from build123d import *

# Parameters (mm, degrees)
SKETCH_1_R      = 1.65
SKETCH_1_R_2    = 1.4
SKETCH_1_R_3    = 1.5
EXTRUDE_1_DEPTH = 4


with BuildPart() as part:
    # 草图1 → 凸台-拉伸1 (new body)
    with BuildSketch(Plane.XY):
        with BuildLine():
            ThreePointArc((-3.477620962, -15.10483871), (0, -19), (3.477620962, -15.10483871))
            ThreePointArc((3.477620962, -15.10483871), (6.883154194, -6.883154194), (15.10483871, -3.477620962))
            ThreePointArc((15.10483871, -3.477620962), (19, 0), (15.10483871, 3.477620962))
            ThreePointArc((15.10483871, 3.477620962), (6.883154194, 6.883154194), (3.477620962, 15.10483871))
            ThreePointArc((3.477620962, 15.10483871), (0, 19), (-3.477620962, 15.10483871))
            ThreePointArc((-3.477620962, 15.10483871), (-6.883154194, 6.883154194), (-15.10483871, 3.477620962))
            ThreePointArc((-15.10483871, 3.477620962), (-19, 0), (-15.10483871, -3.477620962))
            ThreePointArc((-15.10483871, -3.477620962), (-6.883154194, -6.883154194), (-3.477620962, -15.10483871))
        make_face()
        Circle(SKETCH_1_R, mode=Mode.SUBTRACT)
        with Locations((0, -6.5)):
            Circle(SKETCH_1_R_2, mode=Mode.SUBTRACT)
        with Locations((0, 6.5)):
            Circle(SKETCH_1_R_2, mode=Mode.SUBTRACT)
        with Locations((0, -15.5)):
            Circle(SKETCH_1_R_3, mode=Mode.SUBTRACT)
        with Locations((-15.5, 0)):
            Circle(SKETCH_1_R_3, mode=Mode.SUBTRACT)
        with Locations((0, 15.5)):
            Circle(SKETCH_1_R_3, mode=Mode.SUBTRACT)
        with Locations((15.5, 0)):
            Circle(SKETCH_1_R_3, mode=Mode.SUBTRACT)
    extrude(amount=EXTRUDE_1_DEPTH)


solid = part.part
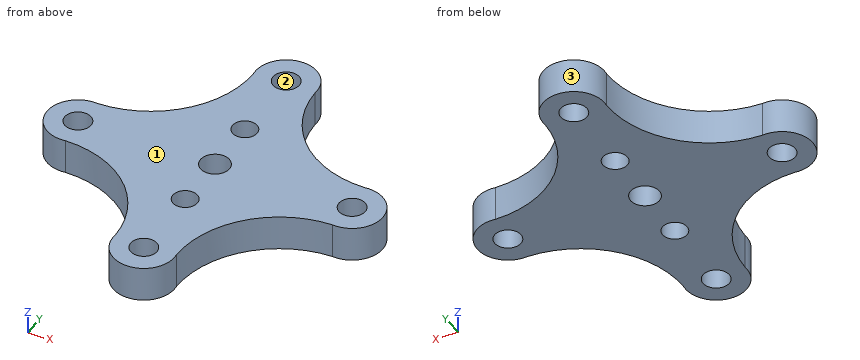
Could you check a few things on this model? Use its own coordinates, in mm. Face numbers are marked on the shaded views. Give positions to 0.01 mm unless a question says otherwise; leave off trailing zeros. Write each loop counter-clockwise with the first axis right and the second up, starting at its lowest first coordinate (ties: lowest second). Pieces come first, ordered by that corner, then holes. Notation, with made-up numbers: (14, 33.25) -> (21, 33.25) arc R14 cw to (21, 55.25) -> close; hole circle Ø7 at (49, 8). An arc over 180 degrees is marked (long way). Answer as CSV lines item,"result". Start each with the question number.
(1) Please list where these lines run through material, in increasing order: line 1 (Y direction, x = 0, z = 2.05); line 2 (X direction, y = -16, z = 0.95); line 3 (X direction, y = 4.5, z = 0.3).
(2) If we section it at B-B, the plane y = 0: Write out the boundary of the cut face in (x, z).
(3) If we section it at C-C, the plane z = 0.85: Write out the boundary of the cut face in (x, y).
(4) If we section it at D-D, the plane y = 6: Write out the boundary of the cut face in (x, z).
(5) I'm going to push flat-ended pins straight in: pin 1 Ø2.5 at (x, y) = (15.5, 0) entering from +Z; pin 2 Ø2 at (y, z) = (-2, 3) entering from -X. Where does each tip first touch, or does it pass through?
(6) If we mould it in two halves opening along X, with no side actions, what happens to the marked faces 1, 2 and 3? For each: +X half, -X half, draft (parallel to the pull), parting line (faces both ways), or undercut.
(7) If we section it at A-A, the plane y = -6.5: Write out the boundary of the cut face in (x, z), and give its area (3 significant figures).
Answer list:
1,line 1,"-19 to -17, -14 to -7.9, -5.1 to -1.65, 1.65 to 5.1, 7.9 to 14, 17 to 19"
1,line 2,"-3.46 to -1.41, 1.41 to 3.46"
1,line 3,"-10.34 to 10.34"
2,outline,"(-19, 0) -> (-17, 0) -> (-17, 4) -> (-19, 4) -> close; (-14, 0) -> (-1.65, 0) -> (-1.65, 4) -> (-14, 4) -> close; (1.65, 0) -> (14, 0) -> (14, 4) -> (1.65, 4) -> close; (17, 0) -> (19, 0) -> (19, 4) -> (17, 4) -> close"
3,outline,"(-15.1, -3.48) arc R11.63 cw to (-3.48, -15.1) arc R3.5 ccw (long way) to (3.48, -15.1) arc R11.63 cw to (15.1, -3.48) arc R3.5 ccw (long way) to (15.1, 3.48) arc R11.63 cw to (3.48, 15.1) arc R3.5 ccw (long way) to (-3.48, 15.1) arc R11.63 cw to (-15.1, 3.48) arc R3.5 ccw (long way) to start; hole circle Ø3 at (-15.5, 0); hole circle Ø3.3 at (0, 0); hole circle Ø3 at (0, -15.5); hole circle Ø3 at (0, 15.5); hole circle Ø2.8 at (0, -6.5); hole circle Ø2.8 at (0, 6.5); hole circle Ø3 at (15.5, 0)"
4,outline,"(-7.87, 0) -> (-1.31, 0) -> (-1.31, 4) -> (-7.87, 4) -> close; (1.31, 0) -> (7.87, 0) -> (7.87, 4) -> (1.31, 4) -> close"
5,pin 1,"through"
5,pin 2,"x = -18.85"
6,face 1,"draft"
6,face 2,"undercut"
6,face 3,"parting line"
7,outline,"(-7.29, 0) -> (-1.4, 0) -> (-1.4, 4) -> (-7.29, 4) -> close; (1.4, 0) -> (7.29, 0) -> (7.29, 4) -> (1.4, 4) -> close"
7,area,"47.1 mm^2"
